Can you work these out from the drawing? Everything is in mm from the part's minimum corner. A direction names the side the tool comes from. Round coordinates to 2 decimals unless told otherwise and drop trailing zeros. Order: outer loops, then holes, each group sorted by start corner. A loop starts at its lowest first (then second) coordinate and runs counter-clockwise, first axis right, second up. Notation, with made-up numbers: M -38.75,-39.5 L -33.75,-39.5 A18 ccw -33.75,-28.5 Z; hole C -9,-37.75 d9. An arc over 180 degrees is marked long. Answer as a JSON object with one key per item and string values. Group by question number.
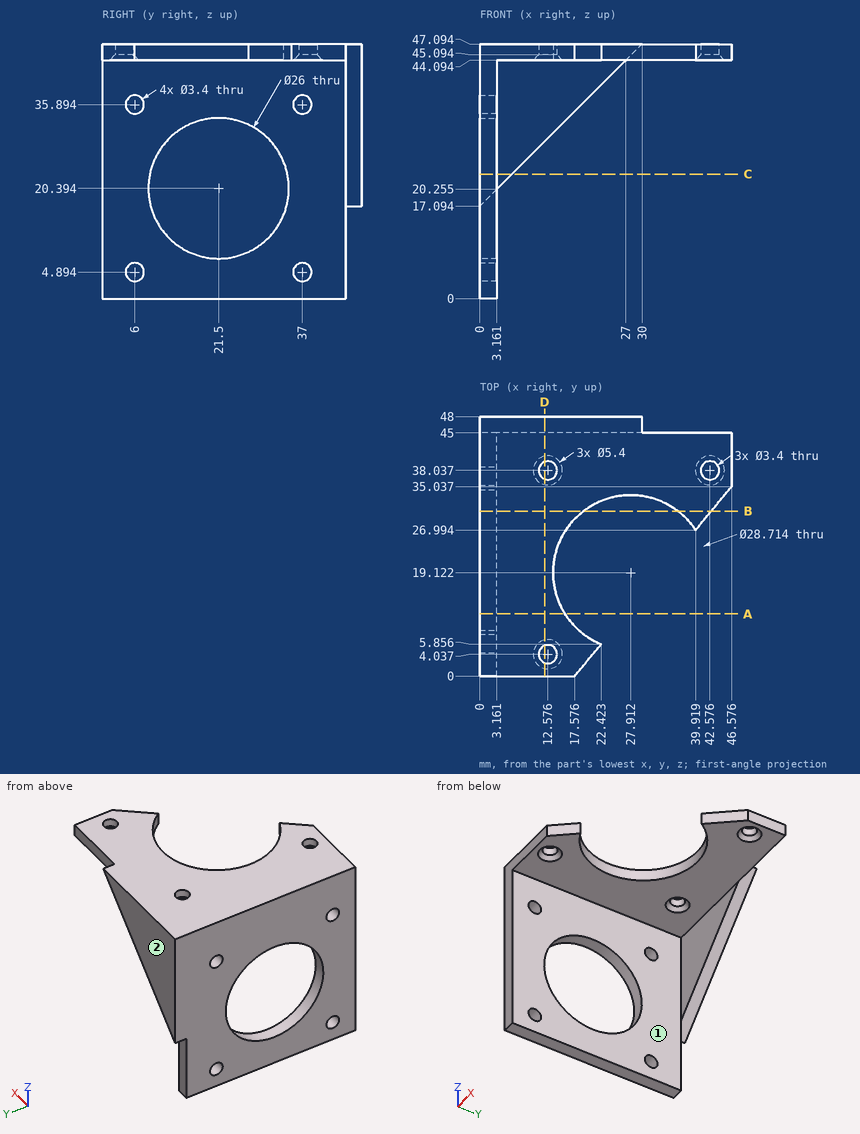
Item 1: Suppose I cut it at C-C, the plane z = 23. Write out the boundary of the cut face in (x, y) (1 decimal).
Item 2: Suppose I cut it at A-A, the plane y = 11.5. Write out the boundary of the cut face in (x, z) (1 decimal).
Item 3: On a 3-axis mill with a long thin cutter (end or side, diameter ignored), from which of +Z, -Z, +X, -X, +Y, -Y can I reach the whole of each face in a straight line? I mean the marked faces 1 and 2. Say none if no direction works.
Item 4: Suppose I cut it at B-B, the plane y = 30.5. Write out the boundary of the cut face in (x, z) (1 decimal), and give its area (3 significant figures).
Item 5: I need wall thicknesses on line 1 (X direction, y = 28, z = 9); line 2 (Y direction, x = 4.5, z = 35.5); line 3 (Z direction, x = 8, y = 12) (1 decimal). Which ranges of each line are inside material? Lowest first, please.
Item 6: Suppose I cut it at D-D, the plane x = 12. State how many separate pieces and enclosed holes the cut face has, and give its area (3 significant figures).
Item 7: I'm going to push flat-ended pins straight in: pin 1 Ø2 at (x, y) = (42.58, 38.04) entering from -Z; pin 2 Ø2.5 at (x, z) = (33.5, 45) entering from +Y; pin 3 Ø22 at (y, z) = (33, 15) entering from +X; pin 4 Ø19 at (x, z) = (15.5, 33.5) entering from -Y. Where does each tip first touch, or does it pass through?
Computed:
{
 "1": {"outline": "M 0,0 L 3.2,0 L 3.2,8.8 L 0,8.8 Z; M 0,34.2 L 3.2,34.2 L 3.2,45 L 5.9,45 L 5.9,48 L 0,48 Z"},
 "2": {"outline": "M 0,0 L 3.2,0 L 3.2,12.1 L 0,12.1 Z; M 0,28.7 L 3.2,28.7 L 3.2,44.1 L 15.7,44.1 L 15.7,47.1 L 0,47.1 Z"},
 "3": {"face 1": "-Z, +X, -Y", "face 2": "+Z, -Z, +X, -X, +Y"},
 "4": {"outline": "M 0,0 L 3.2,0 L 3.2,11 L 0,11 Z; M 0,29.8 L 3.2,29.8 L 3.2,44.1 L 19.2,44.1 L 19.2,47.1 L 0,47.1 Z; M 36.7,44.1 L 42.8,44.1 L 42.8,47.1 L 36.7,47.1 Z", "area": "156 mm^2"},
 "5": {"line 1": "x = 0 to 3.16", "line 2": "y = 45 to 48", "line 3": "z = 44.1 to 47.1"},
 "6": {"separate pieces": "3", "enclosed holes": "0", "area": "168 mm^2"},
 "7": {"pin 1": "passes through", "pin 2": "stops at y = 45", "pin 3": "stops at x = 3.16", "pin 4": "stops at y = 45"}
}
